Build history of the part. All positions in model axes, mm. A direction names the side the tool comes from. Round coordinates to 2 decimals unless told otherwise and drop trailing zeros. Write each loop counter-clockwise with the first axis right and the second up, starting at its lowest first coordinate (ties: lowest second). Pieces come first, ordered by that corner, then holes.
from build123d import *

# Parameters (mm, degrees)
SKETCH_2_W           = 150
SKETCH_2_H           = 43.5
SKETCH_2_R           = 4.5
SKETCH_2_R_2         = 4.05
EXTRUDE_1_DEPTH      = 8
CUT_EXTRUDE_2_DEPTH  = 157.38494173
SKETCH_5_R           = 1.55
CUT_EXTRUDE_3_DEPTH  = 157.38494173
SKETCH_20_R          = 5.5
CUT_EXTRUDE_17_DEPTH = 157.38494173
SKETCH_29_R          = 1.6
CUT_EXTRUDE_18_DEPTH = 157.38494173
CUT_EXTRUDE_5_DEPTH  = 4.5
SKETCH_25_R          = 1.55
CUT_EXTRUDE_13_DEPTH = 157.38494173
CUT_EXTRUDE_11_DEPTH = 2
EXTRUDE_2_DEPTH      = 8


with BuildPart() as part:
    # 草图2 → 凸台-拉伸1 (new body)
    with BuildSketch(Plane.XY):
        with Locations((75, 21.75)):
            Rectangle(SKETCH_2_W, SKETCH_2_H)
        with Locations((10, 8.5)):
            Circle(SKETCH_2_R, mode=Mode.SUBTRACT)
        with Locations((75, 10.5)):
            Circle(SKETCH_2_R_2, mode=Mode.SUBTRACT)
        with Locations((140, 8.5)):
            Circle(SKETCH_2_R, mode=Mode.SUBTRACT)
    extrude_1 = extrude(amount=EXTRUDE_1_DEPTH)

    # 草图4 → 切除-拉伸2 (cut, through all)
    with BuildSketch(Plane(origin=(150, 0, 0), x_dir=(0, 0, -1), z_dir=(1, 0, 0))):
        Polygon((-1.5, 41.7), (-2.5, 41.7), (-2.5, 43.5), (0, 43.5), (0, 38.3), (-1.5, 38.3), align=None)
    cut_extrude_2 = extrude(amount=-CUT_EXTRUDE_2_DEPTH, mode=Mode.SUBTRACT)

    # 草图5 → 切除-拉伸3 (cut, through all)
    with BuildSketch(Plane.XY.offset(8)):
        with Locations((83, 10.5)):
            Circle(SKETCH_5_R)
        with Locations((67, 10.5)):
            Circle(SKETCH_5_R)
    cut_extrude_3 = extrude(amount=-CUT_EXTRUDE_3_DEPTH, mode=Mode.SUBTRACT)

    # 草图20 → 切除-拉伸17 (cut, through all)
    with BuildSketch(Plane(origin=(0, 0, 0), x_dir=(-1, 0, 0), z_dir=(0, 0, -1))):
        with Locations((-75, 10.5)):
            Circle(SKETCH_20_R)
    cut_extrude_17 = extrude(amount=-CUT_EXTRUDE_17_DEPTH, mode=Mode.SUBTRACT)

    # 草图29 → 切除-拉伸18 (cut, through all)
    with BuildSketch(Plane.XY.offset(8)):
        with Locations((22, 8.5)):
            Circle(SKETCH_29_R)
        with Locations(Location((128, 8.5, 0), (0, 0, 180))):
            Circle(SKETCH_29_R)
    cut_extrude_18 = extrude(amount=-CUT_EXTRUDE_18_DEPTH, mode=Mode.SUBTRACT)

    # 草图8 → 切除-拉伸5 (cut)
    with BuildSketch(Plane(origin=(0, 0, 0), x_dir=(-1, 0, 0), z_dir=(0, 0, -1))):
        Polygon((-80.15, 8.854551733), (-80.15, 12.145448267), (-83, 13.790896534), (-85.85, 12.145448267), (-85.85, 8.854551733), (-83, 7.209103466), align=None)
        Polygon((-64.15, 8.854551733), (-64.15, 12.145448267), (-67, 13.790896534), (-69.85, 12.145448267), (-69.85, 8.854551733), (-67, 7.209103466), align=None)
        Polygon((-22, 5.209103466), (-19.15, 6.854551733), (-19.15, 10.145448267), (-22, 11.790896534), (-24.85, 10.145448267), (-24.85, 6.854551733), align=None)
        Polygon((-125.15, 6.854551733), (-125.15, 10.145448267), (-128, 11.790896534), (-130.85, 10.145448267), (-130.85, 6.854551733), (-128, 5.209103466), align=None)
    cut_extrude_5 = extrude(amount=-CUT_EXTRUDE_5_DEPTH, mode=Mode.SUBTRACT)

    # 草图25 → 切除-拉伸13 (cut, through all)
    with BuildSketch(Plane(origin=(0, 0, 0), x_dir=(-1, 0, 0), z_dir=(0, 0, -1))):
        with Locations((-130, 34.5)):
            Circle(SKETCH_25_R)
        with Locations((-20, 34.5)):
            Circle(SKETCH_25_R)
    cut_extrude_13 = extrude(amount=-CUT_EXTRUDE_13_DEPTH, mode=Mode.SUBTRACT)

    # 草图19 → 切除-拉伸11 (cut)
    with BuildSketch(Plane(origin=(0, 0, 2.5), x_dir=(-1, 0, 0), z_dir=(0, 0, -1))):
        with BuildLine():
            Line((-60, 43.5), (-90.247938178, 43.5))
            Line((-90.247938178, 43.5), (-90.247938178, 42.7))
            ThreePointArc((-90.247938178, 42.7), (-89.747938178, 42.2), (-89.247938178, 42.7))
            Line((-89.247938178, 42.7), (-61, 42.7))
            ThreePointArc((-61, 42.7), (-60.5, 42.2), (-60, 42.7))
            Line((-60, 42.7), (-60, 43.5))
        make_face()
    cut_extrude_11 = extrude(amount=-CUT_EXTRUDE_11_DEPTH, mode=Mode.SUBTRACT)

    # 草图22 → 凸台-拉伸2 (add)
    with BuildSketch(Plane.XY.offset(8)):
        with BuildLine():
            Line((0, -3), (4.5, -3))
            ThreePointArc((4.5, -3), (3, -1.5), (4.5, 0))
            Line((4.5, 0), (0, 0))
            ThreePointArc((0, 0), (1.5, -1.5), (0, -3))
        make_face()
        with BuildLine():
            Line((150, 0), (145.5, 0))
            ThreePointArc((145.5, 0), (147, -1.5), (145.5, -3))
            Line((145.5, -3), (150, -3))
            ThreePointArc((150, -3), (148.5, -1.5), (150, 0))
        make_face()
    extrude(amount=-EXTRUDE_2_DEPTH)

    # 镜向2: 凸台-拉伸1, 切除-拉伸2, 切除-拉伸3, 切除-拉伸17, 切除-拉伸18, 切除-拉伸5, 切除-拉伸13, 切除-拉伸11 across plane
    add(extrude_1.mirror(Plane(origin=(0, -1.5, 0), x_dir=(0, 0, 1), z_dir=(0, -1, 0))))
    add(cut_extrude_2.mirror(Plane(origin=(0, -1.5, 0), x_dir=(0, 0, 1), z_dir=(0, -1, 0))), mode=Mode.SUBTRACT)
    add(cut_extrude_3.mirror(Plane(origin=(0, -1.5, 0), x_dir=(0, 0, 1), z_dir=(0, -1, 0))), mode=Mode.SUBTRACT)
    add(cut_extrude_17.mirror(Plane(origin=(0, -1.5, 0), x_dir=(0, 0, 1), z_dir=(0, -1, 0))), mode=Mode.SUBTRACT)
    add(cut_extrude_18.mirror(Plane(origin=(0, -1.5, 0), x_dir=(0, 0, 1), z_dir=(0, -1, 0))), mode=Mode.SUBTRACT)
    add(cut_extrude_5.mirror(Plane(origin=(0, -1.5, 0), x_dir=(0, 0, 1), z_dir=(0, -1, 0))), mode=Mode.SUBTRACT)
    add(cut_extrude_13.mirror(Plane(origin=(0, -1.5, 0), x_dir=(0, 0, 1), z_dir=(0, -1, 0))), mode=Mode.SUBTRACT)
    add(cut_extrude_11.mirror(Plane(origin=(0, -1.5, 0), x_dir=(0, 0, 1), z_dir=(0, -1, 0))), mode=Mode.SUBTRACT)


solid = part.part
1) Wall check: L1, parallel to Y at x = 83, z = 7.15; L2, parallel to Y at x = 20, z = 6; L3, parallel to Y at x = 132.5, z = 6.75. Give the ranges that are in metal, low to high.
Results:
L1: y = -46.5 to -15.05, -11.95 to -3, 0 to 8.95, 12.05 to 43.5
L2: y = -46.5 to -39.05, -35.95 to -3, 0 to 32.95, 36.05 to 43.5
L3: y = -46.5 to -3, 0 to 43.5
2) Slice it at B-B (z = 5.75). Count the separate pieces of the cut face and the enclosed holes in it, plus the area to 3 significant figures.
Results:
separate pieces: 1
enclosed holes: 19
area: 12,500 mm2
3) Which spindle directions (+Z, -Z, +X, -X, +Y, -Y) get a long thin tool onto all of the face, cutting with end or side? Do faces 1 (the flat face through (68.364, 13.003, 2.218)), 2 (the flat face through (76, 40, 1.5)), 3 (the cylindrical face through (20.202, 36.037, 3.944)). Say none if no direction does.
Results:
face 1: -Z
face 2: -Z, +X, -X, +Y
face 3: +Z, -Z
4) Pin check, flat tips, straight feed: pin 1 Ø5 at (x, y) = (83, 10.5) entering from -Z; pin 2 Ø1 at (y, z) = (-23, 2.5) entering from -X; pin 3 Ø1.1 at (x, z) = (69.5, 2) entering from +Y; pin 4 Ø1.6 at (x, z) = (80.5, 3) entering from -Y. Stop position of each tip, or through.
Results:
pin 1: stops at z = 4.5
pin 2: stops at x = 0
pin 3: stops at y = 42.7
pin 4: stops at y = -45.7
5) Slice it at D-D (y = 34.5). Write the cut outline in (x, z), plus the area to 3 significant figures.
Results:
outline: (0, 0) - (18.45, 0) - (18.45, 8) - (0, 8) - close; (21.55, 0) - (128.45, 0) - (128.45, 8) - (21.55, 8) - close; (131.55, 0) - (150, 0) - (150, 8) - (131.55, 8) - close
area: 1,150 mm2
6) Slice it at C-C (x = 33). Write the cut outline in (y, z), plus the area to 3 significant figures.
Results:
outline: (-46.5, 2.5) - (-44.7, 2.5) - (-44.7, 1.5) - (-41.3, 1.5) - (-41.3, 0) - (-3, 0) - (-3, 8) - (-46.5, 8) - close; (0, 0) - (38.3, 0) - (38.3, 1.5) - (41.7, 1.5) - (41.7, 2.5) - (43.5, 2.5) - (43.5, 8) - (0, 8) - close
area: 677 mm2
7) Slice it at A-A (x = 10). Write the cut outline in (y, z), plus the area to 3 significant figures.
Results:
outline: (-46.5, 2.5) - (-44.7, 2.5) - (-44.7, 1.5) - (-41.3, 1.5) - (-41.3, 0) - (-16, 0) - (-16, 8) - (-46.5, 8) - close; (-7, 0) - (-3, 0) - (-3, 8) - (-7, 8) - close; (0, 0) - (4, 0) - (4, 8) - (0, 8) - close; (13, 0) - (38.3, 0) - (38.3, 1.5) - (41.7, 1.5) - (41.7, 2.5) - (43.5, 2.5) - (43.5, 8) - (13, 8) - close
area: 533 mm2
8) Mould opens along X. For faces 4 (the flat face through (24.85, -12, 2)), 5 (the flat face through (0, 21, 4)), 6 (the flat face through (24.85, 9, 2)), 7 (the flat face through (150, 21, 4)) say: released by +X, released by -X, zero draft, split by the parting line, or undercut.
Results:
face 4: undercut
face 5: released by -X
face 6: undercut
face 7: released by +X
